```python
from build123d import *

# Parameters (mm, degrees)
SKETCH1_R      = 4
EXTRUDE1_DEPTH = 140
EXTRUDE2_START = -10
SKETCH2_R      = 4
SKETCH2_R_2    = 2
EXTRUDE2_DEPTH = 10
SKETCH3_R      = 4
SKETCH3_R_2    = 2
EXTRUDE3_DEPTH = 10
CHAMFER1_SIZE  = 0.5


with BuildPart() as part:
    # Sketch1 → Extrude1 (new body)
    with BuildSketch(Plane(origin=(0, 0, 0), x_dir=(1, 0, 0), z_dir=(0, 1, 0))):
        with Locations(Location((0, 0, 0), (0, 0, 270))):
            Circle(SKETCH1_R)
    extrude(amount=EXTRUDE1_DEPTH)

    # Sketch2 → Extrude2 (cut)
    with BuildSketch(Plane(origin=(0, 140, 0), x_dir=(1, 0, 0), z_dir=(0, 1, 0)).offset(EXTRUDE2_START)):
        with Locations(Location((0, 0, 0), (0, 0, 270))):
            Circle(SKETCH2_R)
        with Locations(Location((0, 0, 0), (0, 0, 270))):
            Circle(SKETCH2_R_2, mode=Mode.SUBTRACT)
    extrude(amount=EXTRUDE2_DEPTH, mode=Mode.SUBTRACT)

    # Sketch3 → Extrude3 (cut)
    with BuildSketch(Plane.XZ):
        with Locations(Location((0, 0, 0), (0, 0, 270))):
            Circle(SKETCH3_R)
        with Locations(Location((0, 0, 0), (0, 0, 90))):
            Circle(SKETCH3_R_2, mode=Mode.SUBTRACT)
    extrude(amount=-EXTRUDE3_DEPTH, mode=Mode.SUBTRACT)

    # Chamfer1
    chamfer1_edges = [part.edges().sort_by_distance(p)[0] for p in [
        (0, 0, -2),
        (0, 140, -2),
    ]]
    chamfer(chamfer1_edges, length=CHAMFER1_SIZE)


solid = part.part
```
Can you work these out from the model? Positions are in its coordinate system, mm. A direction names the side the tool comes from. Give positions to 0.01 mm unless a question says otherwise; leave off trailing zeros. Loops run counter-clockwise (first coordinate to the right, second up) from the corner with the lowest first, then second, coordinate; pieces in that order, holes last. Notation, with made-up numbers: M -11.5,39 L 4.5,39 A19 cw 4.5,62 Z; hole C -2.75,31.5 d4. An arc over 180 degrees is marked long. Answer in a Markdown table with one row per item.
1. Suppose I cut it at A-A on z = 0. Write out the boundary of the cut face in (x, y), plus the area to 3 significant figures.
Taken from the geometry:
| item | result |
|---|---|
| outline | M -4,10 L -2,10 L -2,0.5 L -1.5,0 L 1.5,0 L 2,0.5 L 2,10 L 4,10 L 4,130 L 2,130 L 2,139.5 L 1.5,140 L -1.5,140 L -2,139.5 L -2,130 L -4,130 Z |
| area | 1,040 mm² |
2. Suppose I cut it at C-C on y = 41. Write out the boundary of the cut face in (x, z).
Taken from the geometry:
| item | result |
|---|---|
| outline | C 0,0 d8 |
3. Which directions (+Z, -Z, +X, -X, +Y, -Y) give clear straight access to the entire face, cutting with the end or side of a thin tool? Please do faces 1 (the flat face through (-1, 10, 2)), 2 (the flat face through (0, 140, 0)), 3 (the flat face through (-1, 130, -2)).
Taken from the geometry:
| item | result |
|---|---|
| face 1 | -Y |
| face 2 | +Z, -Z, +X, -X, +Y |
| face 3 | +Y |
4. If I drill on line 1 along Y through (x, z) = (2.75, -1); line 2 along X through (y, z) = (34.5, 0.25); line 3 along X through (y, z) = (87.5, -1), over which ranges is the centre line in solid material (lowest first)?
Taken from the geometry:
| item | result |
|---|---|
| line 1 | y = 10 to 130 |
| line 2 | x = -3.99 to 3.99 |
| line 3 | x = -3.87 to 3.87 |
5. Suppose I cut it at B-B on x = 0. Write out the boundary of the cut face in (y, z), plus the area to 3 significant figures.
Taken from the geometry:
| item | result |
|---|---|
| outline | M 0,-1.5 L 0.5,-2 L 10,-2 L 10,-4 L 130,-4 L 130,-2 L 139.5,-2 L 140,-1.5 L 140,1.5 L 139.5,2 L 130,2 L 130,4 L 10,4 L 10,2 L 0.5,2 L 0,1.5 Z |
| area | 1,040 mm² |
6. For pin 1 Ø1 at (x, z) = (-1, 1) entering from -Y; pin 2 Ø1.5 at (x, y) = (2, 111.5) entering from -Z, each with a flat end and sliding along its axis, tell me the tip position at first contact or that it passes through.
Taken from the geometry:
| item | result |
|---|---|
| pin 1 | stops at y = 0 |
| pin 2 | stops at z = -3.8 |
